```python
from build123d import *

# Parameters (mm, degrees)
F0_W     = 200.665613
F0_H     = 24.384
F1_DEPTH = 2.5


with BuildPart() as f1:
    # F0 (on Top) → F1 (new body)
    with BuildSketch(Plane.XY):
        with Locations((86.667197, 0)):
            Rectangle(F0_W, F0_H)
        with BuildLine():
            ThreePointArc((-5.830952, -7.5), (-9.5, 0), (-5.830952, 7.5))
            Line((-5.830952, 7.5), (5.830952, 7.5))
            ThreePointArc((5.830952, 7.5), (9.5, 0), (5.830952, -7.5))
            Line((5.830952, -7.5), (-5.830952, -7.5))
        make_face(mode=Mode.SUBTRACT)
        with BuildLine():
            ThreePointArc((16.169048, -7.5), (12.5, 0), (16.169048, 7.5))
            Line((16.169048, 7.5), (27.830952, 7.5))
            ThreePointArc((27.830952, 7.5), (31.5, 0), (27.830952, -7.5))
            Line((27.830952, -7.5), (16.169048, -7.5))
        make_face(mode=Mode.SUBTRACT)
        with BuildLine():
            ThreePointArc((38.169048, -7.5), (34.5, 0), (38.169048, 7.5))
            Line((38.169048, 7.5), (49.830952, 7.5))
            ThreePointArc((49.830952, 7.5), (53.5, 0), (49.830952, -7.5))
            Line((49.830952, -7.5), (38.169048, -7.5))
        make_face(mode=Mode.SUBTRACT)
        with BuildLine():
            ThreePointArc((60.169048, -7.5), (56.5, 0), (60.169048, 7.5))
            Line((60.169048, 7.5), (71.830952, 7.5))
            ThreePointArc((71.830952, 7.5), (75.5, 0), (71.830952, -7.5))
            Line((71.830952, -7.5), (60.169048, -7.5))
        make_face(mode=Mode.SUBTRACT)
        with BuildLine():
            ThreePointArc((82.169048, -7.5), (78.5, 0), (82.169048, 7.5))
            Line((82.169048, 7.5), (93.830952, 7.5))
            ThreePointArc((93.830952, 7.5), (97.5, 0), (93.830952, -7.5))
            Line((93.830952, -7.5), (82.169048, -7.5))
        make_face(mode=Mode.SUBTRACT)
        with BuildLine():
            ThreePointArc((104.169048, -7.5), (100.5, 0), (104.169048, 7.5))
            Line((104.169048, 7.5), (115.830952, 7.5))
            ThreePointArc((115.830952, 7.5), (119.5, 0), (115.830952, -7.5))
            Line((115.830952, -7.5), (104.169048, -7.5))
        make_face(mode=Mode.SUBTRACT)
        with BuildLine():
            ThreePointArc((126.169048, -7.5), (122.5, 0), (126.169048, 7.5))
            Line((126.169048, 7.5), (137.830952, 7.5))
            ThreePointArc((137.830952, 7.5), (141.5, 0), (137.830952, -7.5))
            Line((137.830952, -7.5), (126.169048, -7.5))
        make_face(mode=Mode.SUBTRACT)
        with BuildLine():
            ThreePointArc((148.169048, -7.5), (144.5, 0), (148.169048, 7.5))
            Line((148.169048, 7.5), (159.830952, 7.5))
            ThreePointArc((159.830952, 7.5), (163.5, 0), (159.830952, -7.5))
            Line((159.830952, -7.5), (148.169048, -7.5))
        make_face(mode=Mode.SUBTRACT)
        with BuildLine():
            ThreePointArc((170.169048, -7.5), (166.5, 0), (170.169048, 7.5))
            Line((170.169048, 7.5), (181.830952, 7.5))
            ThreePointArc((181.830952, 7.5), (185.5, 0), (181.830952, -7.5))
            Line((181.830952, -7.5), (170.169048, -7.5))
        make_face(mode=Mode.SUBTRACT)
    extrude(amount=F1_DEPTH)


solid = f1.part
```
Check sheet for the modelled part. Datum: model origin and axes. Units: mm. Coordinates: 2 decimals unless noted, no trailing zeros. Order: outer loops, then holes, each group sorted by start corner. A loop starts at its lowest first (then second) coordinate and runs counter-clockwise, first axis right, second up. Notation, with made-up numbers: M 5.5,43 L 13.5,43 A9 ccw 13.5,58 Z; hole C 75.5,-7.5 d6. An arc over 180 degrees is marked long. One line per question, with ' | ' between items. Start each with the question number.
Item 1: Sectioned sample at A-A on x = 129. Record the cut outline in (y, z).
Item 2: Sectioned sample at B-B on z = 1.25. Count the separate pieces of the cut face and the enclosed holes in it, and give its area (3 significant figures).
Item 3: Material ranges on line 1 (Y direction, x = 115.5, z = 0.4), recorded low to high.
Item 4: Mould release check, pull along X, two halves, no side actions. Record for faces 1 (the flat face through (85, 8, 0)), 2 (the cylindrical face through (97.5, 0.1, 1.2)): pulls with the +X half, pulls with the -X half, needs draft (parallel to the pull), parting line crosses it, or undercut.
Answer below:
1) outline: M -12.19,0 L -7.5,0 L -7.5,2.5 L -12.19,2.5 Z; M 7.5,0 L 12.19,0 L 12.19,2.5 L 7.5,2.5 Z
2) separate pieces: 1 | enclosed holes: 9 | area: 2,630 mm^2
3) line 1: y = -12.19 to -7.5, 7.5 to 12.19
4) face 1: needs draft | face 2: undercut
